from build123d import *

# Parameters (mm, degrees)
SKETCH1_W           = 35
SKETCH1_H           = 30
BOSS_EXTRUDE1_DEPTH = 22.1
SKETCH2_R           = 3.0875
CUT_EXTRUDE1_DEPTH  = 3
SKETCH3_R           = 1.75
CUT_EXTRUDE2_DEPTH  = 42.682250419
CUT_EXTRUDE3_START  = -3
SKETCH4_R           = 3.0875
CUT_EXTRUDE3_DEPTH  = 3
SKETCH5_R           = 1.75
CUT_EXTRUDE4_DEPTH  = 32.932115495
CUT_EXTRUDE5_DEPTH  = 45.027377846
FILLET1_R           = 0.3
SKETCH7_W           = 35
SKETCH7_H           = 3
CUT_EXTRUDE6_DEPTH  = 10


with BuildPart() as part:
    # Sketch1 → Boss-Extrude1 (new body)
    with BuildSketch(Plane(origin=(0, 0, 0), x_dir=(1, 0, 0), z_dir=(0, 1, 0))):
        Rectangle(SKETCH1_W, SKETCH1_H)
    extrude(amount=BOSS_EXTRUDE1_DEPTH)

    # Sketch2 → Cut-Extrude1 (cut)
    with BuildSketch(Plane(origin=(17.5, 0, 0), x_dir=(0, 0, -1), z_dir=(1, 0, 0))):
        with Locations((0, 12.1)):
            Circle(SKETCH2_R)
    extrude(amount=-CUT_EXTRUDE1_DEPTH, mode=Mode.SUBTRACT)

    # Sketch3 → Cut-Extrude2 (cut, through all)
    with BuildSketch(Plane(origin=(14.5, 0, 0), x_dir=(0, 0, -1), z_dir=(1, 0, 0))):
        with Locations((0, 12.1)):
            Circle(SKETCH3_R)
    extrude(amount=-CUT_EXTRUDE2_DEPTH, mode=Mode.SUBTRACT)

    # Sketch4 → Cut-Extrude3 (cut)
    with BuildSketch(Plane.ZY.offset(17.5).offset(CUT_EXTRUDE3_START)):
        with Locations(Location((0, 12.1, 0), (0, 0, 180))):
            Circle(SKETCH4_R)
    extrude(amount=CUT_EXTRUDE3_DEPTH, mode=Mode.SUBTRACT)

    # Sketch5 → Cut-Extrude4 (cut, through all)
    with BuildSketch(Plane(origin=(0, 22.1, 0), x_dir=(1, 0, 0), z_dir=(0, 1, 0))):
        with Locations(Location((-12.5, 8.5, 0), (0, 0, 270))):
            Circle(SKETCH5_R)
        with Locations(Location((12.5, 8.5, 0), (0, 0, 270))):
            Circle(SKETCH5_R)
        with Locations(Location((12.5, -8.5, 0), (0, 0, 270))):
            Circle(SKETCH5_R)
        with Locations(Location((-12.5, -8.5, 0), (0, 0, 270))):
            Circle(SKETCH5_R)
    extrude(amount=-CUT_EXTRUDE4_DEPTH, mode=Mode.SUBTRACT)

    # Sketch6 → Cut-Extrude5 (cut, through all)
    with BuildSketch(Plane.ZY.offset(17.5)):
        with BuildLine():
            Line((-5, 3), (-5, 13))
            ThreePointArc((-5, 13), (0, 18), (5, 13))
            Line((5, 13), (5, 3))
            Line((5, 3), (15, 3))
            Line((15, 3), (15, 22.1))
            Line((15, 22.1), (-15, 22.1))
            Line((-15, 22.1), (-15, 3))
            Line((-15, 3), (-15, 0))
            Line((-15, 0), (-5, 0))
            Line((-5, 0), (-5, 3))
        make_face()
    extrude(amount=-CUT_EXTRUDE5_DEPTH, mode=Mode.SUBTRACT)

    # Fillet1
    fillet1_edges = [part.edges().sort_by_distance(p)[0] for p in [
        (17.5, 12.1, 3.0875),
        (-17.5, 12.1, 3.0875),
    ]]
    fillet(fillet1_edges, radius=FILLET1_R)

    # Sketch7 → Cut-Extrude6 (cut)
    with BuildSketch(Plane(origin=(0, 3, 0), x_dir=(1, 0, 0), z_dir=(0, 1, 0))):
        with Locations((0, -13.5)):
            Rectangle(SKETCH7_W, SKETCH7_H)
    extrude(amount=-CUT_EXTRUDE6_DEPTH, mode=Mode.SUBTRACT)


solid = part.part
Geometry: final body of the model. Coordinates: model frame, mm. A direction names the side the tool comes from. Give positions to 0.01 mm unless a question says otherwise; leave off trailing zeros. Write each loop counter-clockwise with the first axis right and the second up, starting at its lowest first coordinate (ties: lowest second). Pieces come first, ordered by that corner, then holes.
(1) Cut plane D-D, the plane z = 11.25. Return loops of the section in (x, y).
(2) First-contact query: P1, Ø5, axis at x = -10, y = 7, coming from the +Z side; P2, Ø2, axis at x = 6, z = 9.5, coming from the +Y side; P3, Ø3, axis at y = 12.5, z = -0.5, coming from the +X side. Flat tips, straight axial feed; report the tip coordinate or a pass-through.
(3) Access query for faces 1 (the cylindrical face through (15.87, 15.16, 0.4)), 2 (the flat face through (0, 8, 5)), 3 (the flat face through (0, 6, -5)), 4 (the flat face through (-14.5, 14, 0)). Directions: +Z, -Z, +X, -X, +Y, -Y. A direction counts if a zero-diameter tool reaches every point of the face in a straight line with its end or side. Return the directions, or none.
(4) Ray query, line 1 (X direction, y = 1.05, z = 8.5); line 2 (Y direction, x = 15.8, z = 0); line 3 (Y direction, x = 7, z = 8.75). Return the intervals inside material, ascending.
(5) Cut plane C-C, the plane x = 0.5. Return loops of the section in (y, z), then the cut area to 3 significant figures.
(6) Mould query, pull axis X, two halves, no side actions, for faces 5 (the cylindrical face through (14, 1.5, 9.4)), 6 (the flat face through (-17.5, 7, 2)), 7 (the cylindrical face through (-11, 1.5, 9.4)), 8 (the cylindrical face through (-15.83, 14.84, -1.42)). Classes: released by +X, released by -X, zero draft, split by the parting line, or undercut.
(7) Cut plane A-A, the plane x = 12.5. Return loops of the section in (y, z).
(8) Cut plane B-B, the plane y = 12.1. Return loops of the section in (x, z).
Values follow:
1. outline: (-17.5, 0) - (17.5, 0) - (17.5, 3) - (-17.5, 3) - close
2. P1: stops at z = 5
2. P2: stops at y = 3
2. P3: stops at x = 14.5
3. face 1: +X
3. face 2: +Z, +X, -X, +Y
3. face 3: -Z, +X, -X, +Y, -Y
3. face 4: -X
4. line 1: x = -17.5 to -14.25, -10.75 to 10.75, 14.25 to 17.5
4. line 2: y = 0 to 9.01, 15.19 to 18
4. line 3: y = 0 to 3
5. outline: (0, -5) - (13, -5) arc R5 ccw to (13, 5) - (3, 5) - (3, 12) - (0, 12) - close; hole circle Ø3.5 at (12.1, 0)
5. area: 181 mm2
6. face 5: undercut
6. face 6: released by -X
6. face 7: undercut
6. face 8: zero draft
7. outline: (0, -5) - (13, -5) arc R5 ccw to (13, 5) - (3, 5) - (3, 6.75) - (0, 6.75) - close; (0, 10.25) - (3, 10.25) - (3, 12) - (0, 12) - close; hole circle Ø3.5 at (12.1, 0)
8. outline: (-17.5, -5) - (17.5, -5) - (17.5, -3.39) arc R0.3 ccw to (17.2, -3.09) - (14.5, -3.09) - (14.5, -1.75) - (-14.5, -1.75) - (-14.5, -3.09) - (-17.2, -3.09) arc R0.3 ccw to (-17.5, -3.39) - close; (-17.5, 3.39) arc R0.3 ccw to (-17.2, 3.09) - (-14.5, 3.09) - (-14.5, 1.75) - (14.5, 1.75) - (14.5, 3.09) - (17.2, 3.09) arc R0.3 ccw to (17.5, 3.39) - (17.5, 5) - (-17.5, 5) - close
